Autodesk Inventor part; units mm, degrees
ref_plane "Plano de trabalho1" through (0, 0, 0) normal (0, 0, 1) x (1, 0, 0)
ref_plane "YZ Plane" through (0, 0, 0) normal (1, 0, 0) x (0, 1, 0)
ref_plane "XZ Plane" through (0, 0, 0) normal (0, 1, 0) x (-1, 0, 0)
ref_plane "Plano de trabalho1" through (0, 0, 0) normal (0, 0, 1) x (1, 0, 0)
sketch "Esboço1" plane through (0, 0, 0) normal (0, 0, 1) x (1, 0, 0)
  arc A0 (-40, -30) -> (-30, -40) centre (-30, -30) ccw
  line L0 (30, -40) -> (-30, -40)
  line L1 (40, 30) -> (40, -30)
  arc A1 (40, 30) -> (30, 40) centre (30, 30) ccw
  line L2 (-30, 40) -> (30, 40)
  arc A2 (-30, 40) -> (-40, 30) centre (-30, 30) ccw
  line L3 (-40, -30) -> (-40, 30)
  circle A3 centre (0, 0) radius 5
  circle A4 centre (0, 0) radius 35
  circle A5 centre (30, 30) radius 2
  circle A6 centre (30, -30) radius 2
  circle A7 centre (-30, -30) radius 2
  circle A8 centre (-30, 30) radius 2
  line L4 (0, 0) -> (88.4205, 0)
  circle A9 centre (56.873, 0) radius 9.6
  circle A10 centre (56.873, 0) radius 24.3683
  line L5 (70, -20) -> (70, 13.4311)
  line L6 (0, -54.5393) -> (0, 0)
  line L7 (0, 0) -> (97.6155, 0)
  line L8 (40, -30) -> (40, -40)
  line L9 (40, -40) -> (30, -40)
  line L10 (40, -40) -> (70, -20)
  circle A11 centre (56.873, -14.5) radius 2.1
  point P0 (0, 0)
  point P1 (70, 0)
  point P2 (66.473, 0)
  point P3 (47.273, 0)
  point P4 (5, 0)
  point P5 (0, -5)
  point P6 (0, -40)
  point P7 (35, 0)
  point P8 (0, -35)
  dimension "d0" = 70
  dimension "d3" = 4
  dimension "d4" = 4
  dimension "d5" = 4
  dimension "d6" = 4
  dimension "d7" = 19.2
  dimension "d8" = 30
  dimension "d9" = 20
  dimension "d12" = 4.2
  dimension "d13" = 14.5
  dimension "d14" = 16.873
  dimension "d15" = 16.873
extrude "Extrusão2" add sketch "Esboço1" along normal blind 4 contours L6 A4 A10 L1 L8 L9 L0 | L8 L1 A10 L10 | A4 L4 L1 A10 | A10 L1 L4 A9 L5 L10 picked at (39.1782, -10.8029)
mirror "Espelhamento1" about plane through (70, 0, 0) normal (0, 1, 0) of "Extrusão2"
mirror "Espelhamento2" about plane through (0, 35, 0) normal (-1, 0, 0) of "Extrusão2", "Espelhamento1"
fillet "Arredondamento1" radius 5 8 edges at (40, -40, 2) (70, -20, 2) (70, 20, 2) (40, 40, 2) (-40, 40, 2) (-70, 20, 2) (-70, -20, 2) (-40, -40, 2)
equation "\"d3\" = d6"
equation "\"d4\" = d6"
equation "\"d5\" = d6"
equation "\"d15\" = d14"
properties part number "suporte-superior"
CAD build for the part. Positions are in the model's coordinates, mm. Round coordinates to 2 decimals unless told otherwise and drop trailing zeros. Write each loop counter-clockwise with the first axis right and the second up, starting at its lowest first coordinate (ties: lowest second). Pieces come first, ordered by that corner, then holes. Notation, with made-up numbers: (27, 12.5) -> (83, 12.5) arc R5 cw to (83, 19.5) -> close; hole circle Ø9 at (76, 50.5). An arc over 180 degrees is marked (long way). Answer in a Markdown table with one row per item. Add a question column.
Item 1: Drop flat-ended pins along their axis: pin 1 Ø1.5 at (x, y) = (26.5, 18.5) entering from -Z; pin 2 Ø1.5 at (y, z) = (-22.5, 3) entering from -X. Give the stop position or say it passes through.
Item 2: Saw through at B-B, the plane y = -23. Write the cut outline in (x, z).
Item 3: Saw through at D-D, the plane z = 2.75. Count the separate pieces of the cut face and the enclosed holes in it, then the cut area to 3 significant figures.
Item 4: Saw through at C-C, the plane x = 30. Write the cut outline in (y, z).
Item 5: Drill centre lines: line 1 (X direction, y = -4, z = 1.15); line 2 (X direction, y = 14.5, z = 2.25); line 3 (Y direction, x = -58, z = 1). Where is each one in solid material? Low to high. Write a range as from..to.
Item 6: Mould opens along X. For faces 1 (the face through (69.4, -19.7, 2)), 2 (the face through (-55, -30, 2)), 3 (the face through (-57.842, -16.363, 1.972)) say: pulls with the +X half, pulls with the -X half, needs draft (parallel to the pull), parting line crosses it, or undercut.
Item 7: Saw through at A-A, the plane x = -20. Write the cut outline in (y, z).
Findings below:
| question | item | result |
|---|---|---|
| 1 | pin 1 | passes through |
| 1 | pin 2 | stops at x = -67.37 |
| 2 | outline | (-65.5, 0) -> (-26.38, 0) -> (-26.38, 4) -> (-65.5, 4) -> close; (26.38, 0) -> (65.5, 0) -> (65.5, 4) -> (26.38, 4) -> close |
| 3 | separate pieces | 1 |
| 3 | enclosed holes | 11 |
| 3 | area | 5,460 mm^2 |
| 4 | outline | (-40, 0) -> (-32, 0) -> (-32, 4) -> (-40, 4) -> close; (-28, 0) -> (-18.03, 0) -> (-18.03, 4) -> (-28, 4) -> close; (18.03, 0) -> (28, 0) -> (28, 4) -> (18.03, 4) -> close; (32, 0) -> (40, 0) -> (40, 4) -> (32, 4) -> close |
| 5 | line 1 | x = -70..-65.6, -48.15..-34.77, 34.77..48.15, 65.6..70 |
| 5 | line 2 | x = -70..-58.97, -54.77..-31.86, 31.86..54.77, 58.97..70 |
| 5 | line 3 | y = -28..-16.27, -12.73..-9.53, 9.53..12.73, 16.27..28 |
| 6 | face 1 | pulls with the +X half |
| 6 | face 2 | pulls with the -X half |
| 6 | face 3 | undercut |
| 7 | outline | (-40, 0) -> (-28.72, 0) -> (-28.72, 4) -> (-40, 4) -> close; (28.72, 0) -> (40, 0) -> (40, 4) -> (28.72, 4) -> close |
